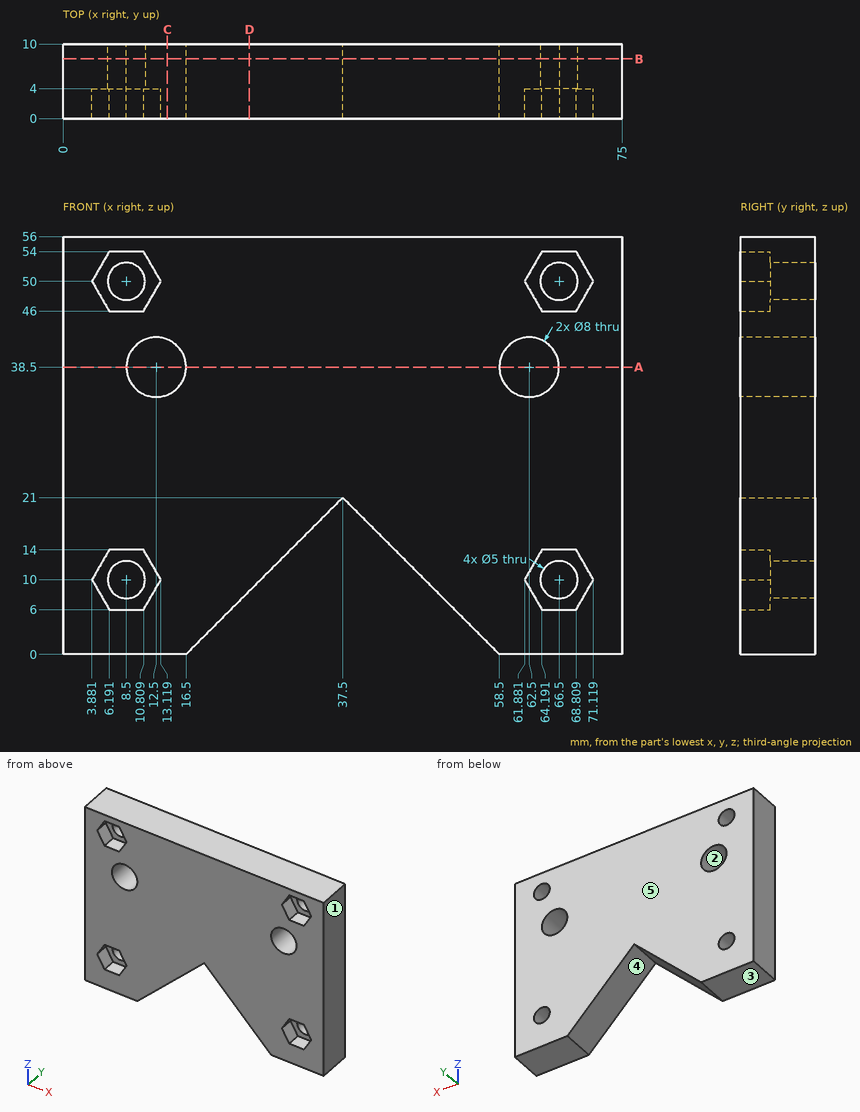
Source: three-view drawing plus pictorial views. Frame: mm from the lowest corner of the part. A direction names the side the tool comes from. Round coordinates to 2 decimals unless told otherwise and drop trailing zeros. Order: outer loops, then holes, each group sorted by start corner. A loop starts at its lowest first (then second) coordinate and runs counter-clockwise, first axis right, second up. Notation, with made-up numbers: (-23, 85.5) - (24, 85.5) arc R17 cw to (24, 97.5) - close; hole circle Ø2 at (-24, 85.5). An arc over 180 degrees is marked (long way). Write each question's results on one line, items separated by ' | '.
Item 1: Section B-B, the plane y = 8. Return the cut outline in (x, z), and give its area (3 significant figures).
Completed:
outline: (0, 0) - (16.5, 0) - (37.5, 21) - (58.5, 0) - (75, 0) - (75, 56) - (0, 56) - close; hole circle Ø5 at (8.5, 10); hole circle Ø5 at (8.5, 50); hole circle Ø8 at (12.5, 38.5); hole circle Ø8 at (62.5, 38.5); hole circle Ø5 at (66.5, 10); hole circle Ø5 at (66.5, 50) | area: 3,580 mm^2
Item 2: Section C-C, the plane x = 14. Return the cut outline in (y, z), and give its area (3 significant figures).
Completed:
outline: (0, 0) - (10, 0) - (10, 34.79) - (0, 34.79) - close; (0, 42.21) - (10, 42.21) - (10, 56) - (0, 56) - close | area: 486 mm^2
Item 3: Material intervals for line 1 along X through (y, z) = (8.25, 38.5); line 2 along Z through (x, y) = (12.5, 6.75); line 3 along Z through (x, y) = (7.5, 7.5), sorted ascending. Write a range as [from, to].
Completed:
line 1: [0, 8.5], [16.5, 58.5], [66.5, 75] | line 2: [0, 34.5], [42.5, 56] | line 3: [0, 7.71], [12.29, 47.71], [52.29, 56]
Item 4: Section A-A, the plane z = 38.5. Return the cut outline in (x, y), and give its area (3 significant figures).
Completed:
outline: (0, 0) - (8.5, 0) - (8.5, 10) - (0, 10) - close; (16.5, 0) - (58.5, 0) - (58.5, 10) - (16.5, 10) - close; (66.5, 0) - (75, 0) - (75, 10) - (66.5, 10) - close | area: 590 mm^2
Item 5: Section D-D, the plane x = 25. Return the cut outline in (y, z).
Completed:
outline: (0, 8.5) - (10, 8.5) - (10, 56) - (0, 56) - close
Item 6: First-contact query: pin 1 Ø1 at (x, y) = (33, 7.5) entering from -Z. Flat tip, straight axial feed; report the tip coordinate or a pass-through.
Completed:
pin 1: z = 16
Item 7: Reachability of the marked faces 4 and 5 from +Z, -Z, +X, -X, +Y, -Y: full face, straight path, thin tool, end or side. Return the list, or none.
Completed:
face 4: -Z, +Y, -Y | face 5: +Z, -Z, +X, -X, +Y
Item 8: Mould query, pull axis Z, two halves, no side actions, for the marked faces 1, 2 and 3. Classes: pulls with the +Z half, pulls with the -Z half, needs draft (parallel to the pull), parting line crosses it, or undercut.
Completed:
face 1: needs draft | face 2: undercut | face 3: pulls with the -Z half
